from build123d import *

# Parameters (mm, degrees)
F0_W     = 67.017666
F0_H     = 52.83216
F1_DEPTH = 25
F2_W     = 18.339222
F2_H     = 46.83216
F3_DEPTH = 20


with BuildPart() as f1:
    # F0 (on Top) → F1 (new body)
    with BuildSketch(Plane.XY):
        Rectangle(F0_W, F0_H)
    extrude(amount=F1_DEPTH)

    # F2 (on face) → F3 (cut)
    with BuildSketch(Plane.XY.offset(25)):
        with Locations((-21.339222, 0)):
            Rectangle(F2_W, F2_H)
        Rectangle(F2_W, F2_H)
        with Locations((21.339222, 0)):
            Rectangle(F2_W, F2_H)
    extrude(amount=-F3_DEPTH, mode=Mode.SUBTRACT)


solid = f1.part
Read the model definition and answer for the solid it produces. Units are mm, in the model's axes. A direction names the side the tool comes from. Round coordinates to 2 decimals unless told otherwise and drop trailing zeros. Write each loop counter-clockwise with the first axis right and the second up, starting at its lowest first coordinate (ties: lowest second). Pieces come first, ordered by that corner, then holes.
1. Determine the mould class of faces 1 (the face through (-21, 23.416, 15)), 2 (the face through (-33.509, 0, 12)), 3 (the face through (33.509, 0, 12)) for opening direction X: pulls with the +X half, pulls with the -X half, needs draft (parallel to the pull), parting line crosses it, or undercut.
2. Given pin 1 Ø9 at (x, y) = (18, 7.5) entering from +Z, flat-ended and moving along its own axis, determine where the tip first touches the part or whether it passes through.
3. The part is cut by section B-B, the plane y = 22.5. Determine the outline of the cut face in (x, z), then the cut area to 3 significant figures.
4. Which of the six approach directions +Z, -Z, +X, -X, +Y, -Y give full straight-line access (tool end or side, diameter ignored) to faces 4 (the face through (0, 0, 0)), 5 (the face through (9.17, 0, 15))?
5. The part is cut by section A-A, the plane x = 24. Determine the outline of the cut face in (y, z).
6. The part is cut by section C-C, the plane z = 19. Determine the outline of the cut face in (x, y), then the cut area to 3 significant figures.
7. Straight lines are drawn through the part: L1, parallel to X at y = -13, z = 12; L2, parallel to Y at x = 7, z = 13; L3, parallel to Z at x = 30, y = 9.5. For each, find the intervals that lie inside material, in ascending order.
Values:
1. face 1: undercut
1. face 2: pulls with the -X half
1. face 3: pulls with the +X half
2. pin 1: stops at z = 5
3. outline: (-33.51, 0) - (33.51, 0) - (33.51, 25) - (30.51, 25) - (30.51, 5) - (12.17, 5) - (12.17, 25) - (9.17, 25) - (9.17, 5) - (-9.17, 5) - (-9.17, 25) - (-12.17, 25) - (-12.17, 5) - (-30.51, 5) - (-30.51, 25) - (-33.51, 25) - close
3. area: 575 mm2
4. face 4: -Z, +X, -X, +Y, -Y
4. face 5: +Z
5. outline: (-26.42, 0) - (26.42, 0) - (26.42, 25) - (23.42, 25) - (23.42, 5) - (-23.42, 5) - (-23.42, 25) - (-26.42, 25) - close
6. outline: (-33.51, -26.42) - (33.51, -26.42) - (33.51, 26.42) - (-33.51, 26.42) - close; hole (-30.51, -23.42) - (-12.17, -23.42) - (-12.17, 23.42) - (-30.51, 23.42) - close; hole (-9.17, -23.42) - (9.17, -23.42) - (9.17, 23.42) - (-9.17, 23.42) - close; hole (12.17, -23.42) - (30.51, -23.42) - (30.51, 23.42) - (12.17, 23.42) - close
6. area: 964 mm2
7. L1: x = -33.51 to -30.51, -12.17 to -9.17, 9.17 to 12.17, 30.51 to 33.51
7. L2: y = -26.42 to -23.42, 23.42 to 26.42
7. L3: z = 0 to 5
